Source: CAD feature listing. Evaluate the final solid. Frame: model axes, mm. A direction names the side the tool comes from. Round coordinates to 2 decimals unless told otherwise and drop trailing zeros. Write each loop counter-clockwise with the first axis right and the second up, starting at its lowest first coordinate (ties: lowest second). Pieces come first, ordered by that corner, then holes. Notation, with made-up numbers: M -32.5,-30 L -5.5,-30 A7 ccw -5.5,-22 Z; hole C 67,67 d4. An arc over 180 degrees is marked long. Put each result on its own line as item: value. Start each with the question number.
```python
from build123d import *

# Parameters (mm, degrees)
F1_DEPTH    = 8
F2_R        = 0.89999
F3_T1_DEPTH = 8


# Not quite as in the source:
# - a fillet or chamfer that OpenCascade refuses, or shapes differently, is made with other operations: its cross-section is extruded or revolved along the edge and cut away or added
# - a fillet or chamfer is up to 0.001 mm smaller than in the source, because OpenCascade refuses the exact size
# - a feature names something its author has since deleted; it is built from what else it names


with BuildPart() as f1:
    # F0 (on Top) → F1 (new body)
    with BuildSketch(Plane.XY):
        with BuildLine():
            ThreePointArc((0, 57), (2.8257898753, 60.2221957995), (6.3892589354, 57.8411618966))
            Line((6.3892589354, 57.8411618966), (8.1279254228, 58.3070361778))
            ThreePointArc((8.1279254228, 58.3070361778), (2.5908427293, 62.0067965499), (-1.8, 57))
            Line((-1.8, 57), (-7.45, 57))
            Line((-7.45, 57), (-7.45, 61.2228588262))
            Line((-7.45, 61.2228588262), (-9.7, 61.2228588262))
            Line((-9.7, 61.2228588262), (-19.05, 61.2228588262))
            Line((-19.05, 61.2228588262), (-19.05, 52.6228588262))
            Line((-19.05, 52.6228588262), (-17.05, 52.6228588262))
            Line((-17.05, 52.6228588262), (-17.05, 40.3365361308))
            Line((-17.05, 40.3365361308), (-11.702219504, 36.2228588262))
            Line((-11.702219504, 36.2228588262), (-16.3474793695, 32.6495820066))
            Line((-16.3474793695, 32.6495820066), (-15.25, 31.2228588262))
            Line((-15.25, 31.2228588262), (-8.75, 36.2228588262))
            Line((-8.75, 36.2228588262), (-15.25, 41.2228588262))
            Line((-15.25, 41.2228588262), (-15.25, 54.4228588262))
            Line((-15.25, 54.4228588262), (-17.25, 54.4228588262))
            Line((-17.25, 54.4228588262), (-17.25, 59.4228588262))
            Line((-17.25, 59.4228588262), (-9.25, 59.4228588262))
            Line((-9.25, 59.4228588262), (-9.25, 57))
            Line((-9.25, 57), (-9.25, 51.4228588262))
            ThreePointArc((-9.25, 51.4228588262), (-3.8052690832, 46.2427536444), (-1.8, 39))
            ThreePointArc((-1.8, 39), (-3.3260618955, 32.624044706), (-7.5735026919, 27.6299564509))
            Line((-7.5735026919, 27.6299564509), (-7.5735026919, 21.0176914536))
            Line((-7.5735026919, 21.0176914536), (-1.8, 11.0176914536))
            Line((-1.8, 11.0176914536), (-1.8, 0))
            ThreePointArc((-1.8, 0), (2.5908427293, -5.0067965499), (8.1279254228, -1.3070361778))
            Line((8.1279254228, -1.3070361778), (6.3892589354, -0.8411618966))
            ThreePointArc((6.3892589354, -0.8411618966), (2.8257898753, -3.2221957995), (0, 0))
            Line((0, 0), (0, 11.5))
            Line((0, 11.5), (-5.7735026919, 21.5))
            Line((-5.7735026919, 21.5), (-5.7735026919, 26.75))
            ThreePointArc((-5.7735026919, 26.75), (-1.5156985287, 32.2288141117), (0, 39))
            Line((0, 39), (0, 57))
        make_face()
        with BuildLine():
            Line((-7.45, 55.2), (-1.8, 55.2))
            Line((-1.8, 55.2), (-1.8, 46.3441924145))
            ThreePointArc((-1.8, 46.3441924145), (-4.2171968015, 49.7784455096), (-7.45, 52.4591018057))
            Line((-7.45, 52.4591018057), (-7.45, 55.2))
        make_face(mode=Mode.SUBTRACT)
    extrude(amount=F1_DEPTH)

    # F2 (radius 0.9 in the source; OpenCascade refuses exactly that, so slightly less here)
    f2_edges = [f1.edges().sort_by_distance(p)[0] for p in [
        (8.127925, 58.307036, 4),
        (6.389259, 57.841162, 4),
        (8.127925, -1.307036, 4),
        (6.389259, -0.841162, 4),
        (-11.70222, 36.222859, 4),
        (-16.347479, 32.649582, 4),
        (-15.25, 31.222859, 4),
        (-8.75, 36.222859, 4),
        (-17.25, 59.422859, 4),
        (-15.25, 54.422859, 4),
        (-9.25, 59.422859, 4),
        (-19.05, 61.222859, 4),
        (-17.05, 52.622859, 4),
        (-9.25, 51.422859, 4),
        (0, 11.5, 4),
        (-7.45, 61.222859, 4),
    ]]
    fillet(f2_edges, radius=F2_R)

    # F3: fillet of radius 3.25 on 2 edges, made by hand

    # F3_s2 → F3_t1 (join)
    with BuildSketch(Plane.XY):
        with BuildLine():
            ThreePointArc((-4.2, 57), (-6.4980970389, 57.9519029611), (-7.45, 60.25))
            Line((-7.45, 60.25), (-7.45, 57))
            Line((-7.45, 57), (-4.2, 57))
        make_face()
        with BuildLine():
            ThreePointArc((-1.3967570543, 58.9774096386), (-2.5946788815, 57.5390574817), (-4.3872442674, 57))
            Line((-4.3872442674, 57), (-1.8, 57))
            ThreePointArc((-1.8, 57), (-1.698162443, 58.0090532384), (-1.3967570543, 58.9774096386))
        make_face()
    extrude(amount=F3_T1_DEPTH)


solid = f1.part
```
(1) Contact query for flat-ended pins moving along their axis: P1, Ø1.4, axis at y = 53.5, z = 5.5, coming from the +X side; P2, Ø6, axis at x = 4.5, y = 8, coming from the -Z side; P3, Ø1.6, axis at y = 24.5, z = 5.5, coming from the +X side; P4, Ø4.5, axis at x = -4.5, z = 2.5, coming from the -Y side. Output: stop coordinate, or through.
(2) Pull-direction query (X, two-part tool) for faces 1 (the flat face through (-15.25, 47, 4)), 2 (the cylindrical face through (3.13, 62.05, 3.94)), 3 (the cylindrical face through (7.75, -1.55, 4.06)), 4 (the flat face through (-13, 61.223, 4)); classes: +X half, -X half, draft (parallel to the pull), parting line (faces both ways), or undercut.
(3) Section query B-B (x = -0.75). Return loops of the section in (y, z), and give its area (3 significant figures).
(4) Section query C-C (x = -3.5). Return loops of the section in (y, z), and give its area (3 significant figures).
(5) Section query A-A (y = 44). Return loops of the section in (x, z).
(6) Section query D-D (y = 9). Return loops of the section in (x, z), and give its area (3 significant figures).
(7) Access query for faces 5 (the cylindrical face through (-1.56, 32.14, 3.94)), 6 (the flat face through (-18.5, 52.623, 3.9)), 7 (the cylindrical face through (-2.534, 57.58, 3.944)), 8 (the cylindrical face through (2.54, -3.17, 3.94)). Directions: +Z, -Z, +X, -X, +Y, -Y. A direction counts if a zero-diameter tool reaches every point of the face in a straight line with its end or side. Return the directions, or none.
(8) Ray query, line 1 along X through (y, z) = (53.5, 7.25); line 2 along X through (y, z) = (48.5, 1.5); line 3 along Y through (x, z) = (-5.5, 1). Return the intervals inside material, ascending.
Entries:
1. P1: x = 0
1. P2: through
1. P3: x = -5.77
1. P4: y = 11.8
2. face 1: undercut
2. face 2: undercut
2. face 3: +X half
2. face 4: draft
3. outline: M -3.08,0 L 12.8,0 L 12.8,8 L -3.08,8 Z; M 34.18,0 L 60.08,0 L 60.08,8 L 34.18,8 Z
3. area: 334 mm2
4. outline: M 13.96,0 L 17.56,0 L 17.56,8 L 13.96,8 Z; M 29.05,0 L 32.29,0 L 32.29,8 L 29.05,8 Z; M 45.71,0 L 48.95,0 L 48.95,8 L 45.71,8 Z; M 55.2,0 L 57.12,0 L 57.12,8 L 55.2,8 Z
4. area: 96.0 mm2
5. outline: M -17.05,0 L -15.25,0 L -15.25,8 L -17.05,8 Z; M -2.72,0 L 0,0 L 0,8 L -2.72,8 Z
6. outline: M -1.8,0 L 0,0 L 0,8 L -1.8,8 Z
6. area: 14.4 mm2
7. face 5: +Z, -Z, +X
7. face 6: +Z, -Z, -X, -Y
7. face 7: +Z, -Z, +Y
7. face 8: +Z, -Z
8. line 1: -19.05 to -15.25, -9.25 to -7.45, -1.8 to 0
8. line 2: -17.05 to -15.25, -5.49 to -3.15, -1.8 to 0
8. line 3: 17.43 to 21.03, 26.98 to 29.49, 48.51 to 51.02, 55.2 to 57.27
